The drawing under review shows one solid part. Ordinate dimensions are in mm from its lowest x, y, z. A direction names the side the tool comes from. Give positions to 0.01 mm unless a question says otherwise; leave off trailing zeros. Loops run counter-clockwise (first coordinate to the right, second up) from the corner with the lowest first, then second, coordinate; pieces in that order, holes last. Notation, with made-up numbers: M 81,-10 L 136,-10 A36 cw 136,27 Z; hole C 19,49 d4. An arc over 180 degrees is marked long. Answer as CSV lines item,"result".
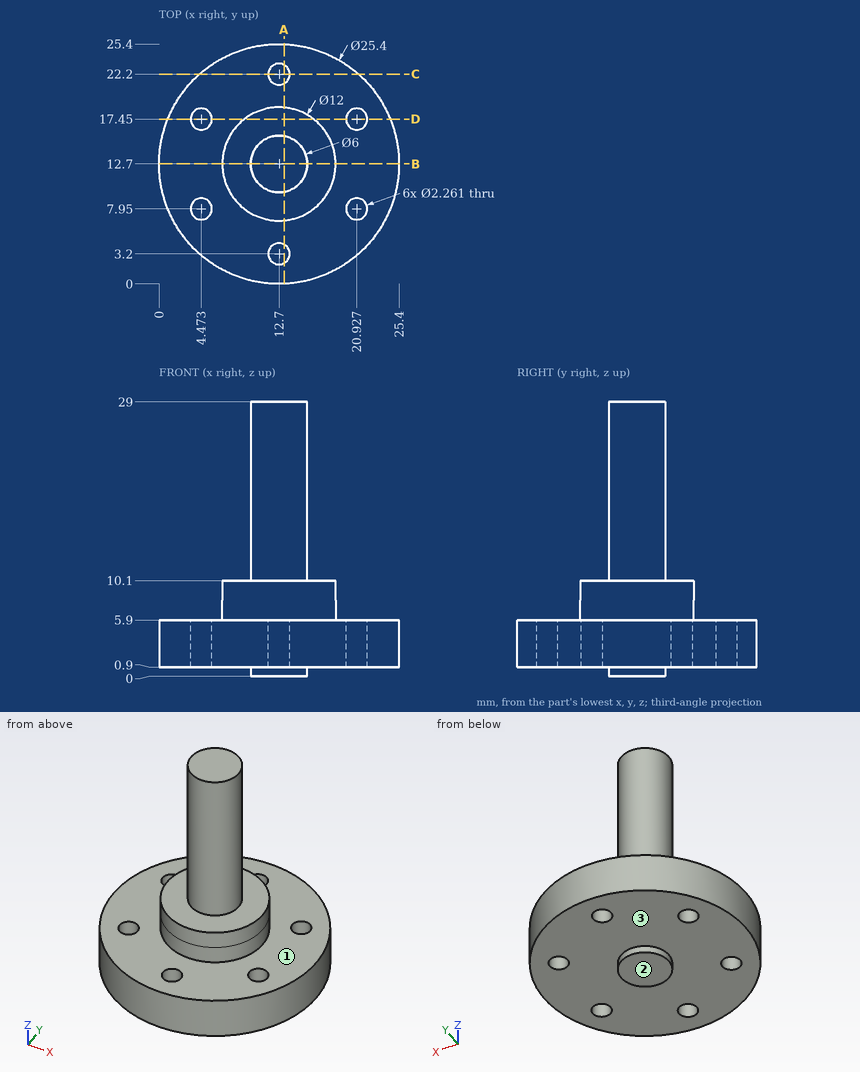
1. We need section B-B, the plane y = 12.7. Write out the cut boundary in (x, z), plus the area to 3 significant figures.
Answer block:
outline,"M 0,0.9 L 9.7,0.9 L 9.7,0 L 15.7,0 L 15.7,0.9 L 25.4,0.9 L 25.4,5.9 L 18.7,5.9 L 18.7,10.1 L 15.7,10.1 L 15.7,29 L 9.7,29 L 9.7,10.1 L 6.7,10.1 L 6.7,5.9 L 0,5.9 Z"
area,"296 mm²"
2. We need section A-A, the plane x = 13.25. Write out the cut boundary in (y, z) (1 decimal).
Answer block:
outline,"M 0,0.9 L 2.2,0.9 L 2.2,5.9 L 0,5.9 Z; M 4.2,0.9 L 9.8,0.9 L 9.8,0 L 15.6,0 L 15.6,0.9 L 21.2,0.9 L 21.2,5.9 L 18.7,5.9 L 18.7,10.1 L 15.6,10.1 L 15.6,29 L 9.8,29 L 9.8,10.1 L 6.7,10.1 L 6.7,5.9 L 4.2,5.9 Z; M 23.2,0.9 L 25.4,0.9 L 25.4,5.9 L 23.2,5.9 Z"
3. We need section C-C, the plane y = 22.2. Write out the cut boundary in (x, z).
Answer block:
outline,"M 4.27,0.9 L 11.57,0.9 L 11.57,5.9 L 4.27,5.9 Z; M 13.83,0.9 L 21.13,0.9 L 21.13,5.9 L 13.83,5.9 Z"
4. For the marked faces 1, 2 and 3, list the 3-axis set-ups (+Z, -Z, +X, -X, +Y, -Y) from which the entire face can be reached by the end or side of a thin tool; tool diameter is ignored.
Answer block:
face 1,"+Z"
face 2,"-Z, +X, -X, +Y, -Y"
face 3,"-Z"
5. For P1, Ø6, axis at x = 21, y = 17.5, coming from the +Z side; P2, Ø1.8, axis at x = 4.47, y = 7.95, coming from the -Z side; P3, Ø8, axis at x = 10, y = 11, coming from the +Z side; P4, Ø12, axis at y = 10, z = 15, coming from the +X side, all flat-tipped, find the tip position at first contact; note any pin that passes through.
Answer block:
P1,"z = 5.9"
P2,"through"
P3,"z = 29"
P4,"x = 18.7"
6. To check wall thickness, follow L1, parallel to Y at x = 12.7, z = 2.3; L2, parallel to Z at x = 2, y = 9.5; L3, parallel to Z at x = 15.5, y = 14.25. State the ranges of each line that lie inside material, in increasing order. Write a range as [from, to].
Answer block:
L1,"[0, 2.07], [4.33, 21.07], [23.33, 25.4]"
L2,"[0.9, 5.9]"
L3,"[0.9, 10.1]"
7. We need section D-D, the plane y = 17.45. Write out the cut boundary in (x, z) (1 decimal).
Answer block:
outline,"M 0.9,0.9 L 3.3,0.9 L 3.3,5.9 L 0.9,5.9 Z; M 5.6,0.9 L 19.8,0.9 L 19.8,5.9 L 16.4,5.9 L 16.4,10.1 L 9,10.1 L 9,5.9 L 5.6,5.9 Z; M 22.1,0.9 L 24.5,0.9 L 24.5,5.9 L 22.1,5.9 Z"
